Geometry: final body of the model. Coordinates: model frame, mm. Give positions to 0.01 mm unless a question says otherwise; leave off trailing zeros. Answer in a Markdown table with one row per item.
from build123d import *

# Parameters (mm, degrees)
SKETCH_1_R               = 23.74347741
EXTRUDE_1_DEPTH          = 3
CUT_EXTRUDE_1_DEPTH      = 294.143309663
CUT_EXTRUDE_1_DEPTH_BACK = 294.143309663
SKETCH_2_R               = 2.5
CUT_EXTRUDE_2_DEPTH      = 294.143309663
CUT_EXTRUDE_2_DEPTH_BACK = 294.143309663
SKETCH_3_R               = 1.5
CUT_EXTRUDE_3_DEPTH      = 294.143309663
CUT_EXTRUDE_3_DEPTH_BACK = 294.143309663
SKETCH_4_R               = 10.25
CUT_EXTRUDE_4_DEPTH      = 294.143309663
CUT_EXTRUDE_4_DEPTH_BACK = 294.143309663
SKETCH_5_R               = 1.5
CUT_EXTRUDE_5_DEPTH      = 294.143309663
CUT_EXTRUDE_5_DEPTH_BACK = 294.143309663
SKETCH_6_R               = 1.5
CUT_EXTRUDE_6_DEPTH      = 294.143309663
CUT_EXTRUDE_6_DEPTH_BACK = 294.143309663
SKETCH_7_R               = 1.5


with BuildPart() as part:
    # 草图1 → 凸台-拉伸1 (new body)
    with BuildSketch(Plane.XY):
        with BuildLine():
            Line((44.764783638, 38.458868953), (4.334015044, 74.86289651))
            ThreePointArc((4.334015044, 74.86289651), (-1.881238093, 78.67160853), (-9.048597084, 80))
            Line((-9.048597084, 80), (-225.951402916, 80))
            ThreePointArc((-225.951402916, 80), (-233.118761907, 78.67160853), (-239.334015044, 74.86289651))
            Line((-239.334015044, 74.86289651), (-279.764783638, 38.458868953))
            ThreePointArc((-279.764783638, 38.458868953), (-281.748934241, 33.886916076), (-279.593885752, 29.392989871))
            ThreePointArc((-279.593885752, 29.392989871), (-276.958783906, 25.06173547), (-277.521429039, 20.023188369))
            ThreePointArc((-277.521429039, 20.023188369), (-282, 0), (-277.521429039, -20.023188369))
            ThreePointArc((-277.521429039, -20.023188369), (-276.958783906, -25.06173547), (-279.593885752, -29.392989871))
            ThreePointArc((-279.593885752, -29.392989871), (-281.657387183, -32.949868258), (-280.946152423, -37))
            Line((-280.946152423, -37), (-274.883974596, -47.5))
            ThreePointArc((-274.883974596, -47.5), (-269.393593539, -52.990381057), (-261.893593539, -55))
            Line((-261.893593539, -55), (26.893593539, -55))
            ThreePointArc((26.893593539, -55), (34.393593539, -52.990381057), (39.883974596, -47.5))
            Line((39.883974596, -47.5), (45.946152423, -37))
            ThreePointArc((45.946152423, -37), (46.657387183, -32.949868258), (44.593885752, -29.392989871))
            ThreePointArc((44.593885752, -29.392989871), (41.958783906, -25.06173547), (42.521429039, -20.023188369))
            ThreePointArc((42.521429039, -20.023188369), (47, 0), (42.521429039, 20.023188369))
            ThreePointArc((42.521429039, 20.023188369), (41.958783906, 25.06173547), (44.593885752, 29.392989871))
            ThreePointArc((44.593885752, 29.392989871), (46.748934241, 33.886916076), (44.764783638, 38.458868953))
        make_face()
        Circle(SKETCH_1_R, mode=Mode.SUBTRACT)
        with Locations((-235, 0)):
            Circle(SKETCH_1_R, mode=Mode.SUBTRACT)
    extrude(amount=EXTRUDE_1_DEPTH)

    # 草图2 → 切除-拉伸1 (cut, two sides: drawn at the far end of the back side and taken through both)
    with BuildSketch(Plane(origin=(0, 0, 0), x_dir=(-1, 0, 0), z_dir=(0, 0, -1)).offset(-CUT_EXTRUDE_1_DEPTH_BACK)):
        with Locations((40.75, -34)):
            Circle(SKETCH_2_R)
        with Locations((40.75, 34)):
            Circle(SKETCH_2_R)
        with Locations((-40.75, 34)):
            Circle(SKETCH_2_R)
        with Locations((-40.75, -34)):
            Circle(SKETCH_2_R)
        with Locations((275.75, -34)):
            Circle(SKETCH_2_R)
        with Locations((275.75, 34)):
            Circle(SKETCH_2_R)
        with Locations((194.25, 34)):
            Circle(SKETCH_2_R)
        with Locations((194.25, -34)):
            Circle(SKETCH_2_R)
    extrude(amount=CUT_EXTRUDE_1_DEPTH + CUT_EXTRUDE_1_DEPTH_BACK, mode=Mode.SUBTRACT)

    # 草图3 → 切除-拉伸2 (cut, two sides: drawn at the far end of the back side and taken through both)
    with BuildSketch(Plane.XY.offset(3).offset(-CUT_EXTRUDE_2_DEPTH_BACK)):
        with Locations((-251.264045876, 39.264880132)):
            Circle(SKETCH_3_R)
        with Locations((-274.264880132, 16.264045876)):
            Circle(SKETCH_3_R)
        with Locations((-274.264880132, -16.264045876)):
            Circle(SKETCH_3_R)
        with Locations((-251.264045876, -39.264880132)):
            Circle(SKETCH_3_R)
        with Locations((-218.735954124, 39.264880132)):
            Circle(SKETCH_3_R)
        with Locations((-195.735119868, 16.264045876)):
            Circle(SKETCH_3_R)
        with Locations((-195.735119868, -16.264045876)):
            Circle(SKETCH_3_R)
        with Locations((-218.735954124, -39.264880132)):
            Circle(SKETCH_3_R)
        with Locations((-16.264045876, -39.264880132)):
            Circle(SKETCH_3_R)
        with Locations((-39.264880132, -16.264045876)):
            Circle(SKETCH_3_R)
        with Locations((-39.264880132, 16.264045876)):
            Circle(SKETCH_3_R)
        with Locations((-16.264045876, 39.264880132)):
            Circle(SKETCH_3_R)
        with Locations((16.264045876, 39.264880132)):
            Circle(SKETCH_3_R)
        with Locations((39.264880132, 16.264045876)):
            Circle(SKETCH_3_R)
        with Locations((39.264880132, -16.264045876)):
            Circle(SKETCH_3_R)
        with Locations((16.264045876, -39.264880132)):
            Circle(SKETCH_3_R)
        with BuildLine():
            Line((-239.500175319, -39.468321754), (-239.500178729, -40.236009311))
            ThreePointArc((-239.500178729, -40.236009311), (-239.099568481, -41.256477718), (-238.111715855, -41.731863382))
            ThreePointArc((-238.111715855, -41.731863382), (-235.000000357, -41.847714357), (-231.888284858, -41.731863435))
            ThreePointArc((-231.888284858, -41.731863435), (-230.900432223, -41.256477788), (-230.499821958, -40.236009387))
            Line((-230.499821958, -40.236009387), (-230.499825355, -39.468321831))
            ThreePointArc((-230.499825355, -39.468321831), (-230.378047604, -38.781085812), (-230.027538462, -38.177540862))
            ThreePointArc((-230.027538462, -38.177540862), (-234.999999671, 38.5), (-239.97246219, -38.177540777))
            ThreePointArc((-239.97246219, -38.177540777), (-239.621953058, -38.781085733), (-239.500175319, -39.468321754))
        make_face()
        with BuildLine():
            Line((-4.500175319, -39.468321754), (-4.500178729, -40.236009311))
            ThreePointArc((-4.500178729, -40.236009311), (-4.099568481, -41.256477718), (-3.111715855, -41.731863382))
            ThreePointArc((-3.111715855, -41.731863382), (-3.57e-07, -41.847714357), (3.111715142, -41.731863435))
            ThreePointArc((3.111715142, -41.731863435), (4.099567777, -41.256477788), (4.500178042, -40.236009387))
            Line((4.500178042, -40.236009387), (4.500174645, -39.468321831))
            ThreePointArc((4.500174645, -39.468321831), (4.621952396, -38.781085812), (4.972461538, -38.177540862))
            ThreePointArc((4.972461538, -38.177540862), (3.29e-07, 38.5), (-4.97246219, -38.177540777))
            ThreePointArc((-4.97246219, -38.177540777), (-4.621953058, -38.781085733), (-4.500175319, -39.468321754))
        make_face()
    extrude(amount=CUT_EXTRUDE_2_DEPTH + CUT_EXTRUDE_2_DEPTH_BACK, mode=Mode.SUBTRACT)

    # 草图4 → 切除-拉伸3 (cut, two sides: drawn at the far end of the back side and taken through both)
    with BuildSketch(Plane(origin=(0, 0, 0), x_dir=(-1, 0, 0), z_dir=(0, 0, -1)).offset(-CUT_EXTRUDE_3_DEPTH_BACK)):
        with Locations((225.951402916, 60)):
            Circle(SKETCH_4_R)
        with Locations((9.048597084, 60)):
            Circle(SKETCH_4_R)
        with Locations((117.5, -35)):
            Circle(SKETCH_4_R)
        with Locations((117.5, 60)):
            Circle(SKETCH_4_R)
    extrude(amount=CUT_EXTRUDE_3_DEPTH + CUT_EXTRUDE_3_DEPTH_BACK, mode=Mode.SUBTRACT)

    # 草图5 → 切除-拉伸4 (cut, two sides: drawn at the far end of the back side and taken through both)
    with BuildSketch(Plane.XY.offset(3).offset(-CUT_EXTRUDE_4_DEPTH_BACK)):
        with Locations((-134, -24.75)):
            Circle(SKETCH_5_R)
        with Locations((-134, -45.25)):
            Circle(SKETCH_5_R)
        with Locations((-101, -45.25)):
            Circle(SKETCH_5_R)
        with Locations((-101, -24.75)):
            Circle(SKETCH_5_R)
    extrude(amount=CUT_EXTRUDE_4_DEPTH + CUT_EXTRUDE_4_DEPTH_BACK, mode=Mode.SUBTRACT)

    # 草图6 → 切除-拉伸5 (cut, two sides: drawn at the far end of the back side and taken through both)
    with BuildSketch(Plane.XY.offset(3).offset(-CUT_EXTRUDE_5_DEPTH_BACK)):
        with Locations((-209.951402916, 76)):
            Circle(SKETCH_6_R)
        with Locations((-209.951402916, 60)):
            Circle(SKETCH_6_R)
        with Locations((-215.871834176, 48.891341485)):
            Circle(SKETCH_6_R)
        with Locations((-231.685290109, 74.937286824)):
            Circle(SKETCH_6_R)
        with Locations((-248.547809826, 61.184227506)):
            Circle(SKETCH_6_R)
        with Locations((-239.229232955, 52.329375962)):
            Circle(SKETCH_6_R)
        with Locations((4.229232955, 52.329375962)):
            Circle(SKETCH_6_R)
        with Locations((-19.128165824, 48.891341485)):
            Circle(SKETCH_6_R)
        with Locations((-25.048597084, 60)):
            Circle(SKETCH_6_R)
        with Locations((-25.048597084, 76)):
            Circle(SKETCH_6_R)
        with Locations((-3.314709891, 74.937286824)):
            Circle(SKETCH_6_R)
        with Locations((13.547809826, 61.184227506)):
            Circle(SKETCH_6_R)
    extrude(amount=CUT_EXTRUDE_5_DEPTH + CUT_EXTRUDE_5_DEPTH_BACK, mode=Mode.SUBTRACT)

    # 草图7 → 切除-拉伸6 (cut, two sides: drawn at the far end of the back side and taken through both)
    with BuildSketch(Plane.XY.offset(3).offset(-CUT_EXTRUDE_6_DEPTH_BACK)):
        with Locations((-134, 49.75)):
            Circle(SKETCH_7_R)
        with Locations((-134, 70.25)):
            Circle(SKETCH_7_R)
        with Locations((-101, 70.25)):
            Circle(SKETCH_7_R)
        with Locations((-101, 49.75)):
            Circle(SKETCH_7_R)
    extrude(amount=CUT_EXTRUDE_6_DEPTH + CUT_EXTRUDE_6_DEPTH_BACK, mode=Mode.SUBTRACT)


solid = part.part
Q1. First-contact query: pin 1 (3 mm diameter, centred on x = -275.75, y = -34, fed in from -Z); pin 2 (0.6 mm diameter, centred on y = -40, z = 2, fed in from +X); pin 3 (1 mm diameter, centred on y = 6.5, z = 2, fed in from -X). Flat tips, straight axial feed; report the tip coordinate or a pass-through.
Check values:
| item | result |
|---|---|
| pin 1 | through |
| pin 2 | x = 44.39 |
| pin 3 | x = -281.62 |
Q2. Material intervals for line 1 along X through (y, z) = (1, 2.95); line 2 along Y through (x, z) = (-117.5, 0.9); line 3 along X through (y, z) = (8, 0.2), sorted ascending.
Check values:
| item | result |
|---|---|
| line 1 | -281.99 to -273.49, -196.51 to -38.49, 38.49 to 46.99 |
| line 2 | -55 to -45.25, -24.75 to 49.75, 70.25 to 80 |
| line 3 | -281.31 to -272.66, -197.34 to -37.66, 37.66 to 46.31 |
Q3. Draft query along Y for faces 1 (the flat face through (-259.266, 56.916, 1.479)), 2 (the cylindrical face through (-269.489, -52.935, 1.479)), 3 (the cylindrical face through (-215.71, 60.45, 1.52)). Return one class per face: pulls with the +Y half, pulls with the -Y half, needs draft (parallel to the pull), parting line crosses it, or undercut.
Check values:
| item | result |
|---|---|
| face 1 | pulls with the +Y half |
| face 2 | pulls with the -Y half |
| face 3 | undercut |
Q4. Cut plane A-A (z = 2). Give the number of separate pieces and of enclosed holes in the cut face, and give its area (3 significant figures).
Check values:
| item | result |
|---|---|
| separate pieces | 1 |
| enclosed holes | 50 |
| area | 30,600 mm² |
